Work out the finished part from the listing and answer in its coordinate system (mm). A direction names the side the tool comes from. Give positions to 0.01 mm unless a question says otherwise; leave off trailing zeros. Order: outer loops, then holes, each group sorted by start corner. A loop starts at its lowest first (then second) coordinate and runs counter-clockwise, first axis right, second up. Notation, with made-up numbers: (77, -2) -> (91, -2) arc R15 cw to (91, 23) -> close; hole circle Ø11 at (54.25, 13). An arc over 180 degrees is marked (long way). Answer as CSV lines item,"result". Start each with the question number.
1. A cutting plane is placed at B-B (x = 0). Give the vertices of the cut face in (y, z).
2. Find the intervals of material crossed by L1, parallel to Z at x = -16.4, y = 5; L2, parallel to Y at x = -17.3, z = 9.3; L3, parallel to X at y = 4.5, z = -19, in increasing order.
3. For faces 1 (the flat face through (-15.05, 5, -4)), 2 (the flat face through (2.26, 2.25, 16.81)), 3 (the flat face through (-17, 5, -22)), 4 (the cylindrical face through (-4.347, 5.055, 19.699)), 5 (the cylindrical face through (-17.069, 5.608, -14.634)), determine the directions among +Z, -Z, +X, -X, +Y, -Y from which every point of the face is accessible in a straight line to the end or side of a thin tool.
4. A cutting plane is placed at C-C (y = 8.75). Give the vertices of the cut face in (x, z) (3 decimals).
5. For a pull along Y with two mould halves and no side action, classify faces 6 (the flat face through (3.709, 9.746, 16.88)), 7 (the flat face through (-7, 0, 18)), 8 (the cylindrical face through (-17.07, 6.41, 10.03)) as released by +Y, released by -Y, zero draft, split by the parting line, or undercut.
6. Flat-ended cylindrical pins translate along their axes: pin 1 (12 mm diameter, centred on x = -13, z = 7.5, fed in from +Y); pin 2 (4 mm diameter, centred on y = 5, z = -16.1, fed in from -X); pin 3 (3 mm diameter, centred on y = 5, z = 9.3, fed in from -X); pin 4 (4 mm diameter, centred on x = 10, y = 5, fed in from -Z). Find the tip coordinate at first contact, or state that the pin passes through.
7. A cutting plane is placed at D-D (z = -7.5). Give the vertices of the cut face in (x, y), then the cut area to 4 significant figures.
from build123d import *
from OCP.BRepFilletAPI import BRepFilletAPI_MakeChamfer

# Parameters (mm, degrees)
SKETCH1_W                             = 38.1
SKETCH1_H                             = 44
BOSS_EXTRUDE1_DEPTH                   = 10
CUT_EXTRUDE1_REACH                    = 32.772
SKETCH2_W                             = 34.1
SKETCH2_H                             = 37.65
F_1_8_0_125_DIAMETER_HOLE1_AT_2_COUNT = 2
F_1_8_0_125_DIAMETER_HOLE1_AT_2_PITCH = 25.4
DRAFT1_ANGLE                          = 3
CUT_EXTRUDE2_DEPTH                    = 33.229580472
CUT_EXTRUDE3_DEPTH                    = 45.389768844
FILLET2_R                             = 3.175
CHAMFER1_SIZE                         = 0.5
CHAMFER2_SIZE                         = 0.5
CHAMFER2_SIZE2                        = 0.528377251


with BuildPart() as part:
    # Sketch1 → Boss-Extrude1 (new body)
    with BuildSketch(Plane(origin=(0, 0, 0), x_dir=(1, 0, 0), z_dir=(0, 1, 0))):
        Rectangle(SKETCH1_W, SKETCH1_H)
    extrude(amount=BOSS_EXTRUDE1_DEPTH)

    # Sketch2 → Cut-Extrude1 (cut, up to next)
    with BuildSketch(Plane(origin=(0, 10, 0), x_dir=(1, 0, 0), z_dir=(0, 1, 0)), mode=Mode.PRIVATE) as cut_extrude1_sk1:
        with Locations((2, 3.175)):
            Rectangle(SKETCH2_W, SKETCH2_H)
    cut_extrude1_tool1 = extrude(cut_extrude1_sk1.sketch, amount=-CUT_EXTRUDE1_REACH, mode=Mode.PRIVATE) & part.part
    add(cut_extrude1_tool1.solids().sort_by_distance((2, 10, -3.175))[0], mode=Mode.SUBTRACT)

    # Sketch3 → 1/8 (0.125) Diameter Hole1 (revolve, cut)
    with BuildSketch(Plane(origin=(-19.05, 5, -16.1), x_dir=(0, 0, 1), z_dir=(0, 1, 0))):
        Polygon((0, 0), (0, 4), (2.2225, 4), (1.5875, 3.365), (1.5875, 0.635), (2.2225, 0), align=None)
    f_1_8_0_125_diameter_hole1 = revolve(axis=Axis((-25.4, 5, -16.1), (1, 0, 0)), mode=Mode.SUBTRACT)

    # 1/8 (0.125) Diameter Hole1 at 2: 1/8 (0.125) Diameter Hole1 ×2
    with Locations(*[(0, 0, i * F_1_8_0_125_DIAMETER_HOLE1_AT_2_PITCH) for i in range(1, F_1_8_0_125_DIAMETER_HOLE1_AT_2_COUNT)]):
        add(f_1_8_0_125_diameter_hole1, mode=Mode.SUBTRACT)

    # Draft1
    draft1_faces = [part.faces().sort_by_distance(p)[0] for p in [
        (0, 5, 22),
    ]]
    draft(draft1_faces, Plane(origin=(-19.05, 10, 22), x_dir=(0, 0, -1), z_dir=(-1, 0, 0)), DRAFT1_ANGLE)

    # Sketch7 → Cut-Extrude2 (cut, through all)
    with BuildSketch(Plane(origin=(0, 10, 0), x_dir=(1, 0, 0), z_dir=(0, 1, 0))):
        Polygon((-15.05, -15.65), (19.05, -15.65), (19.05, -17.437105274), align=None)
    extrude(amount=-CUT_EXTRUDE2_DEPTH, mode=Mode.SUBTRACT)

    # Sketch8 → Cut-Extrude3 (cut, through all)
    with BuildSketch(Plane(origin=(-0.859157962, 0, 16.393710517), x_dir=(-0.9986295347545739, 0, -0.05233595624294398), z_dir=(0.05233595624294399, 0, -0.998629534754574))):
        with BuildLine():
            Line((-7.189683217, 7.5), (0.810316783, 7.5))
            ThreePointArc((0.810316783, 7.5), (3.310316783, 5), (0.810316783, 2.5))
            Line((0.810316783, 2.5), (-7.189683217, 2.5))
            ThreePointArc((-7.189683217, 2.5), (-9.689683217, 5), (-7.189683217, 7.5))
        make_face()
    extrude(amount=-CUT_EXTRUDE3_DEPTH, mode=Mode.SUBTRACT)

    # Fillet2
    fillet2_edges = [part.edges().sort_by_distance(p)[0] for p in [
        (-15.05, 5, 15.65),
    ]]
    fillet(fillet2_edges, radius=FILLET2_R)

    # Chamfer1
    chamfer1_edges = [part.edges().sort_by_distance(p)[0] for p in [
        (8.817245881, 5, 16.900829354),
        (2.326153905, 2.5, 16.560645639),
        (-4.164938071, 5, 16.220461923),
        (2.326153905, 7.5, 16.560645639),
    ]]
    chamfer(chamfer1_edges, length=CHAMFER1_SIZE)

    # Chamfer2: one chamfer whose edges measure the first distance from different faces: ONE call of the kernel's chamfer builder (chamfer() names one face for all edges)
    chamfer2_edges_1 = [part.edges().sort_by_distance(p)[0] for p in [
        (-15.05, 0, -4.68148125),
        (-15.05, 5, -22),
        (-15.05, 10, -4.68148125),
        (3.504416669, 10, 16.622395774),
        (3.504416669, 0, 16.622395774),
        (-14.178063628, 10, 14.822563279),
        (-14.178063628, 0, 14.822563279),
    ]]
    chamfer2_edges_2 = [part.edges().sort_by_distance(p)[0] for p in [
        (19.05, 5, 17.437105274),
    ]]
    chamfer2_side_2 = [part.faces().sort_by_distance(p)[0] for p in [
        (9.643116423, 5, 16.944111395),
    ]]
    chamfer2 = BRepFilletAPI_MakeChamfer(part.part.solid().wrapped)
    for e in chamfer2_edges_1:
        chamfer2.Add(CHAMFER2_SIZE, e.wrapped)
    for e in chamfer2_edges_2:
        chamfer2.Add(CHAMFER2_SIZE, CHAMFER2_SIZE2, e.wrapped, chamfer2_side_2[0].wrapped)  # the first distance lies on this face
    add(Compound.cast(chamfer2.Shape()), mode=Mode.REPLACE)


solid = part.part
Answer sheet:
1,outline,"(0, 16.94) -> (0.5, 16.44) -> (2, 16.44) -> (2.5, 16.94) -> (2.5, 23) -> (0, 23) -> close; (7.5, 16.94) -> (8, 16.44) -> (9.5, 16.44) -> (10, 16.94) -> (10, 23) -> (7.5, 23) -> close"
2,L1,"z = -22 to -17.69, -14.51 to 7.71, 10.89 to 22.14"
2,L2,"y = 0 to 3.41, 6.59 to 10"
2,L3,"x = -19.05 to -15.05"
3,face 1,"-Z, +X, +Y, -Y"
3,face 2,"-Z"
3,face 3,"-Z, +X, -X, +Y, -Y"
3,face 4,"+Z"
3,face 5,"+X, -X"
4,outline,"(-19.05, -22) -> (-15.55, -22) -> (-15.05, -21.5) -> (-15.05, 12.637) arc R3.175 cw to (-12.041, 15.808) -> (18.551, 17.411) -> (19.05, 17.965) -> (19.05, 23.997) -> (-19.05, 22) -> close"
5,face 6,"released by +Y"
5,face 7,"released by -Y"
5,face 8,"undercut"
6,pin 1,"stops at y = 10"
6,pin 2,"stops at x = -18.83"
6,pin 3,"passes through"
6,pin 4,"stops at z = 16.9"
7,outline,"(-19.05, 0) -> (-15.55, 0) -> (-15.05, 0.5) -> (-15.05, 9.5) -> (-15.55, 10) -> (-19.05, 10) -> close"
7,area,"39.75 mm^2"
